Check sheet for the modelled part. Datum: model origin and axes. Units: mm. A direction names the side the tool comes from. Coordinates: 2 decimals unless noted, no trailing zeros. Loops run counter-clockwise (first coordinate to the right, second up) from the corner with the lowest first, then second, coordinate; pieces in that order, holes last. Notation, with made-up numbers: M -20.5,41 L 24.5,41 A27 ccw 24.5,68 Z; hole C 43,-22.5 d8. An arc over 180 degrees is marked long. Use CSV: the item, a comma, the result in double quotes. Start each with the question number.
(1) Section check A-A on z = -3. Record the cut outline in (x, y), and give its area (3 significant figures).
(2) Section check C-C on y = -0.5. Give the number of separate pieces and of enclosed holes in the cut face, and give its area (3 significant figures).
(3) Draft check along X on faces 1 (the cylindrical face through (18.859, -0.021, -18.797)), 2 (the flat face through (0, 0, 20)), 3 (the cylindrical face through (-10.07, 0.02, 10.12)). Enter one of: pulls with the +X half, pulls with the -X half, needs draft (parallel to the pull), parting line crosses it, or undercut.
(4) Section check D-D on x = 9. Record the cut outline in (y, z).
(5) Set-up check for faces 4 (the flat face through (9.11, 0.02, 6.92)), 5 (the flat face through (9, -1.5, 0)): record each of +Z, -Z, +X, -X, +Y, -Y from which the full face is reachable in a straight line by a thin tool's end or side.
(6) Go/stop test with a flat-tipped pin: pin 1 Ø2.5 at (x, z) = (16, 16) entering from -Y. Record where the tip stops, or that it passes through.
(7) Section check B-B on x = 2. Record the cut outline in (y, z).
(8) Scan lines: line 1 (X direction, y = -0.8, z = -16); line 2 (X direction, y = 0.05, z = -17). Record each from-to range of solid material in increasing order.
from build123d import *

# Parameters (mm, degrees)
SKETCH1_W           = 40
SKETCH1_H           = 40
BOSS_EXTRUDE1_DEPTH = 1.5
FILLET1_R           = 4
SKETCH3_R           = 7
SKETCH3_R_2         = 1.55
CUT_EXTRUDE2_DEPTH  = 3


with BuildPart() as part:
    # Sketch1 → Boss-Extrude1 (new body, symmetric)
    with BuildSketch(Plane(origin=(0, 0, 0), x_dir=(1, 0, 0), z_dir=(0, 1, 0))):
        Rectangle(SKETCH1_W, SKETCH1_H)
    extrude(amount=BOSS_EXTRUDE1_DEPTH, both=True)

    # Fillet1
    fillet1_edges = [part.edges().sort_by_distance(p)[0] for p in [
        (20, 0, 20),
        (-20, 0, 20),
        (-20, 0, -20),
        (20, 0, -20),
    ]]
    fillet(fillet1_edges, radius=FILLET1_R)

    # Sketch3 → Cut-Extrude2 (cut)
    with BuildSketch(Plane(origin=(0, 1.5, 0), x_dir=(1, 0, 0), z_dir=(0, 1, 0))):
        Circle(SKETCH3_R)
        with BuildLine():
            Line((5.903984489, -8.096015511), (7.903984489, -10.096015511))
            ThreePointArc((7.903984489, -10.096015511), (10.096015511, -10.096015511), (10.096015511, -7.903984489))
            Line((10.096015511, -7.903984489), (8.096015511, -5.903984489))
            ThreePointArc((8.096015511, -5.903984489), (5.903984489, -5.903984489), (5.903984489, -8.096015511))
        make_face()
        with Locations((16, -16)):
            Circle(SKETCH3_R_2)
        with BuildLine():
            ThreePointArc((-7.903984489, -10.096015511), (-10.096015511, -10.096015511), (-10.096015511, -7.903984489))
            Line((-10.096015511, -7.903984489), (-8.096015511, -5.903984489))
            ThreePointArc((-8.096015511, -5.903984489), (-5.903984489, -5.903984489), (-5.903984489, -8.096015511))
            Line((-5.903984489, -8.096015511), (-7.903984489, -10.096015511))
        make_face()
        with BuildLine():
            Line((-5.903984489, 8.096015511), (-7.903984489, 10.096015511))
            ThreePointArc((-7.903984489, 10.096015511), (-10.096015511, 10.096015511), (-10.096015511, 7.903984489))
            Line((-10.096015511, 7.903984489), (-8.096015511, 5.903984489))
            ThreePointArc((-8.096015511, 5.903984489), (-5.903984489, 5.903984489), (-5.903984489, 8.096015511))
        make_face()
        with Locations((-16, 16)):
            Circle(SKETCH3_R_2)
        with BuildLine():
            ThreePointArc((7.903984489, 10.096015511), (10.096015511, 10.096015511), (10.096015511, 7.903984489))
            Line((10.096015511, 7.903984489), (8.096015511, 5.903984489))
            ThreePointArc((8.096015511, 5.903984489), (5.903984489, 5.903984489), (5.903984489, 8.096015511))
            Line((5.903984489, 8.096015511), (7.903984489, 10.096015511))
        make_face()
        with Locations((16, 16)):
            Circle(SKETCH3_R_2)
        with Locations((-16, -16)):
            Circle(SKETCH3_R_2)
        with BuildLine():
            ThreePointArc((-6, 5.815728072), (-5.903984489, 5.903984489), (-5.815728072, 6))
            Line((-5.815728072, 6), (-6, 6))
            Line((-6, 6), (-6, 5.815728072))
        make_face()
        with BuildLine():
            Line((-6, -6), (-5.815728072, -6))
            ThreePointArc((-5.815728072, -6), (-5.903984489, -5.903984489), (-6, -5.815728072))
            Line((-6, -5.815728072), (-6, -6))
        make_face()
        with BuildLine():
            Line((6, -6), (6, -5.815728072))
            ThreePointArc((6, -5.815728072), (5.903984489, -5.903984489), (5.815728072, -6))
            Line((5.815728072, -6), (6, -6))
        make_face()
        with BuildLine():
            ThreePointArc((5.815728072, 6), (5.903984489, 5.903984489), (6, 5.815728072))
            Line((6, 5.815728072), (6, 6))
            Line((6, 6), (5.815728072, 6))
        make_face()
        with BuildLine():
            ThreePointArc((-6, 3.605551275), (-7, 0), (-6, -3.605551275))
            Line((-6, -3.605551275), (-6, 3.605551275))
        make_face()
        with BuildLine():
            Line((-3.605551275, 6), (3.605551275, 6))
            ThreePointArc((3.605551275, 6), (0, 7), (-3.605551275, 6))
        make_face()
        with BuildLine():
            Line((6, 3.605551275), (6, -3.605551275))
            ThreePointArc((6, -3.605551275), (6.745368782, -1.870828693), (7, 0))
            ThreePointArc((7, 0), (6.745368782, 1.870828693), (6, 3.605551275))
        make_face()
        with BuildLine():
            ThreePointArc((-3.605551275, -6), (0, -7), (3.605551275, -6))
            Line((3.605551275, -6), (-3.605551275, -6))
        make_face()
    extrude(amount=-CUT_EXTRUDE2_DEPTH, mode=Mode.SUBTRACT)


solid = part.part
Outcome:
1,outline,"M -20,-1.5 L -6.32,-1.5 L -6.32,1.5 L -20,1.5 Z; M 6.32,-1.5 L 20,-1.5 L 20,1.5 L 6.32,1.5 Z"
1,area,"82.1 mm²"
2,separate pieces,"1"
2,enclosed holes,"9"
2,area,"1,340 mm²"
3,face 1,"pulls with the +X half"
3,face 2,"needs draft"
3,face 3,"undercut"
4,outline,"M -1.5,-20 L 1.5,-20 L 1.5,-10.55 L -1.5,-10.55 Z; M -1.5,-6.81 L 1.5,-6.81 L 1.5,6.81 L -1.5,6.81 Z; M -1.5,10.55 L 1.5,10.55 L 1.5,20 L -1.5,20 Z"
5,face 4,"+Y, -Y"
5,face 5,"+Z, -Z, +X, -X, -Y"
6,pin 1,"passes through"
7,outline,"M -1.5,-20 L 1.5,-20 L 1.5,-6.71 L -1.5,-6.71 Z; M -1.5,6.71 L 1.5,6.71 L 1.5,20 L -1.5,20 Z"
8,line 1,"x = -20 to -17.55, -14.45 to 14.45, 17.55 to 20"
8,line 2,"x = -19.87 to -17.18, -14.82 to 14.82, 17.18 to 19.87"
